```python
from build123d import *

# Parameters (mm, degrees)
SKETCH1_R            = 2
BOSS_EXTRUDE1_DEPTH  = 1.2
SKETCH2_R            = 1.3
BOSS_EXTRUDE2_DEPTH  = 1.6
SKETCH3_R            = 2
BOSS_EXTRUDE3_DEPTH  = 42.2
SKETCH4_R            = 3
BOSS_EXTRUDE4_DEPTH  = 18
BOSS_EXTRUDE7_DEPTH  = 2.4
SKETCH6_W            = 6.9
SKETCH6_H            = 10
BOSS_EXTRUDE8_DEPTH  = 1.2
BOSS_EXTRUDE9_DEPTH  = 10
CHAMFER1_SIZE        = 1
BOSS_EXTRUDE10_DEPTH = 4.85
SKETCH9_W            = 6.9
SKETCH9_H            = 9.7
BOSS_EXTRUDE11_DEPTH = 1
SKETCH11_W           = 4.5
SKETCH11_H           = 1.55
CUT_EXTRUDE1_DEPTH   = 1


with BuildPart() as part:
    # Sketch1 → Boss-Extrude1 (new body)
    with BuildSketch(Plane(origin=(0, 0, 0), x_dir=(0, 0, -1), z_dir=(1, 0, 0))):
        Circle(SKETCH1_R)
    extrude(amount=BOSS_EXTRUDE1_DEPTH)

    # Sketch2 → Boss-Extrude2 (add)
    with BuildSketch(Plane(origin=(1.2, 0, 0), x_dir=(0, 0, -1), z_dir=(1, 0, 0))):
        Circle(SKETCH2_R)
    extrude(amount=BOSS_EXTRUDE2_DEPTH)

    # Sketch3 → Boss-Extrude3 (add)
    with BuildSketch(Plane(origin=(2.8, 0, 0), x_dir=(0, 0, -1), z_dir=(1, 0, 0))):
        Circle(SKETCH3_R)
    extrude(amount=BOSS_EXTRUDE3_DEPTH)

    # Sketch4 → Boss-Extrude4 (add)
    with BuildSketch(Plane(origin=(45, 0, 0), x_dir=(0, 0, -1), z_dir=(1, 0, 0))):
        Circle(SKETCH4_R)
    extrude(amount=BOSS_EXTRUDE4_DEPTH)

    # Sketch5 → Boss-Extrude7 (add)
    with BuildSketch(Plane.ZY.offset(-45)):
        with BuildLine():
            ThreePointArc((3, 0), (2.598076211, 1.5), (1.5, 2.598076211))
            Line((1.5, 2.598076211), (1.5, -2.598076211))
            ThreePointArc((1.5, -2.598076211), (2.598076211, -1.5), (3, 0))
        make_face()
        with BuildLine():
            Line((-1.5, -2.598076211), (-1.5, 2.598076211))
            ThreePointArc((-1.5, 2.598076211), (-3, 0), (-1.5, -2.598076211))
        make_face()
    extrude(amount=BOSS_EXTRUDE7_DEPTH)

    # Sketch6 → Boss-Extrude8 (add)
    with BuildSketch(Plane(origin=(63, 0, 0), x_dir=(0, 0, -1), z_dir=(1, 0, 0))):
        Rectangle(SKETCH6_W, SKETCH6_H)
    extrude(amount=BOSS_EXTRUDE8_DEPTH)

    # Sketch7 → Boss-Extrude9 (add)
    with BuildSketch(Plane.ZY.offset(-63)):
        Polygon((-3.45, 5), (-3.45, 9), (-2.25, 9), (-2.25, -9), (-3.45, -9), (-3.45, -5), align=None)
        Polygon((3.45, 9), (2.25, 9), (2.25, -9), (3.45, -9), (3.45, -5), (3.45, 5), align=None)
    extrude(amount=-BOSS_EXTRUDE9_DEPTH)

    # Chamfer1
    chamfer1_edges = [part.edges().sort_by_distance(p)[0] for p in [
        (73, 9, -2.85),
        (73, -9, -2.85),
        (73, -9, 2.85),
        (73, 9, 2.85),
    ]]
    chamfer(chamfer1_edges, length=CHAMFER1_SIZE)

    # Sketch8 → Boss-Extrude10 (add, symmetric)
    with BuildSketch(Plane(origin=(0, 0, 0), x_dir=(1, 0, 0), z_dir=(0, 1, 0))):
        Polygon((63, 3.45), (66, 3.45), (65, 6.25), (64, 6.25), align=None)
        Polygon((68, 6.25), (69, 6.25), (70, 3.45), (67, 3.45), align=None)
        Polygon((72, 6.25), (73, 6.25), (74, 3.45), (71, 3.45), align=None)
    boss_extrude10 = extrude(amount=BOSS_EXTRUDE10_DEPTH, both=True)

    # Mirror1: Boss-Extrude10 across plane
    add(boss_extrude10.mirror(Plane.XY))

    # Sketch9 → Boss-Extrude11 (add)
    with BuildSketch(Plane(origin=(73, 0, 0), x_dir=(0, 0, -1), z_dir=(1, 0, 0))):
        Rectangle(SKETCH9_W, SKETCH9_H)
    extrude(amount=BOSS_EXTRUDE11_DEPTH)

    # Sketch11 → Cut-Extrude1 (cut)
    with BuildSketch(Plane(origin=(74, 0, 0), x_dir=(0, 0, -1), z_dir=(1, 0, 0))):
        with Locations((0, -4.075)):
            Rectangle(SKETCH11_W, SKETCH11_H)
        with Locations((0, 4.075)):
            Rectangle(SKETCH11_W, SKETCH11_H)
    extrude(amount=-CUT_EXTRUDE1_DEPTH, mode=Mode.SUBTRACT)


solid = part.part
```
Can you work these out from the model? Positions are in its coordinate system, mm. A direction names the side the tool comes from. Give positions to 0.01 mm unless a question says otherwise; leave off trailing zeros. Loops run counter-clockwise (first coordinate to the right, second up) from the corner with the lowest first, then second, coordinate; pieces in that order, holes last. Notation, with made-up numbers: M 16,13.25 L 39,13.25 A14 cw 39,27.25 Z; hole C -35,80 d3. An arc over 180 degrees is marked long. Use one line per item in the form item = value. Start each with the question number.
(1) On a 3-axis mill with a long thin cutter (end or side, diameter ignored), from which of +Z, -Z, +X, -X, +Y, -Y can I reach the whole of each face in a straight line? I mean faces 4 (the flat face through (66.8, -0.1, 3.45)), 5 (the flat face through (69, -4.85, 5)), 6 (the cylindrical face through (1.99, 1.29, 0.17)), 7 (the flat face through (73, 6, 3)), 8 (the flat face through (69, 4.85, 5)). Say none if no direction works.
(2) Thinking about a two-plate mould opening in Z: for faces 1 (the flat face through (63.507, -0.068, -4.87)), 2 (the flat face through (0, 0, 0)), 3 (the flat face through (64, -5, 0)), which applies, released by +Z, released by -Z, zero draft, split by the parting line, or undercut?
(3) I want a section at D-D, the plane z = 4.5. Write out the boundary of the cut face in (x, y) (3 decimals), and give its area (3 significant figures).
(4) I want a section at C-C, the plane x = 24.5. Write out the boundary of the cut face in (y, z).
(5) I want a section at B-B, the plane z = -4.25. Write out the boundary of the cut face in (x, y).
(6) I'm going to push flat-ended pins straight in: P1, Ø0.9, axis at x = 73, z = -3.5, coming from the -Y side; P2, Ø0.5, axis at x = 73.5, z = 0, coming from the -Y side; P3, Ø10, axis at x = 36, y = -1.5, coming from the -Z side. Where does each tip first touch, or does it pass through?
(7) Please list where these lines run through material, in increasing order: line 1 (X direction, y = -4, z = -3.75); line 2 (Z direction, x = 66.5, y = -7.5); line 3 (X direction, y = 2.75, z = 1.5).
(8) I want a section at A-A, the plane z = 0. Write out the boundary of the cut face in (x, y).
Worked out:
q1.face_4 = +Z
q1.face_5 = +Z, +X, -X, -Y
q1.face_6 = none
q1.face_7 = +Z, -Z, +X, +Y
q1.face_8 = +Z, +X, -X, +Y
q2.face_1 = released by -Z
q2.face_2 = zero draft
q2.face_3 = undercut
q3.outline = M 63.375,-4.85 L 65.625,-4.85 L 65.625,4.85 L 63.375,4.85 Z; M 67.375,-4.85 L 69.625,-4.85 L 69.625,4.85 L 67.375,4.85 Z; M 71.375,-4.85 L 73.625,-4.85 L 73.625,4.85 L 71.375,4.85 Z
q3.area = 65.5 mm²
q4.outline = C 0,0 d4
q5.outline = M 63.29,-4.85 L 65.71,-4.85 L 65.71,4.85 L 63.29,4.85 Z; M 67.29,-4.85 L 69.71,-4.85 L 69.71,4.85 L 67.29,4.85 Z; M 71.29,-4.85 L 73.71,-4.85 L 73.71,4.85 L 71.29,4.85 Z
q6.P1 = -8.45
q6.P2 = -3.3
q6.P3 = -2
q7.line_1 = 63.11 to 65.89, 67.11 to 69.89, 71.11 to 73.89
q7.line_2 = -3.45 to -2.25, 2.25 to 3.45
q7.line_3 = 63 to 64.2, 73 to 74
q8.outline = M 0,-2 L 1.2,-2 L 1.2,-1.3 L 2.8,-1.3 L 2.8,-2 L 45,-2 L 45,-3 L 63,-3 L 63,-5 L 64.2,-5 L 64.2,5 L 63,5 L 63,3 L 45,3 L 45,2 L 2.8,2 L 2.8,1.3 L 1.2,1.3 L 1.2,2 L 0,2 Z; M 73,-3.3 L 74,-3.3 L 74,3.3 L 73,3.3 Z
